Check sheet for the modelled part. Datum: model origin and axes. Units: mm. A direction names the side the tool comes from. Round coordinates to 2 decimals unless told otherwise and drop trailing zeros. Loops run counter-clockwise (first coordinate to the right, second up) from the corner with the lowest first, then second, coordinate; pieces in that order, holes last. Notation, with made-up numbers: (2, 87) - (31, 87) arc R17 cw to (31, 116) - close; hole circle Ø6 at (75, 74). An arc over 180 degrees is marked (long way). Put each result on its own line as item: value. Start each with the question number.
Item 1: Tool access check on faces 1 (the flat face through (-12.24, 16.91, 0.49)), 2 (the flat face through (2, 3, 1)), 3 (the cylindrical face through (-8.962, -15.834, 0.493)), 4 (the flat face through (-10.633, 19.445, 0.986)). Record the directions out of +Z, -Z, +X, -X, +Y, -Y that give a thin tool (end or side, any length) a straight path to the whole face; none if there is none.
Item 2: Section check B-B, the plane z = 0.35. Record the cut outline in (x, y).
Item 3: Draft check along X on faces 5 (the flat face through (2, -2, 0)), 6 (the flat face through (-10.656, -19.462, 0.986)), 7 (the cylindrical face through (-12.09, 19.06, 0.99)). Enter one of: pulls with the +X half, pulls with the -X half, needs draft (parallel to the pull), parting line crosses it, or undercut.
Item 4: Section check A-A, the plane x = 3. Record the cut outline in (y, z).
Item 5: Section check D-D, the plane y = -12. Record the cut outline in (x, z), and give its area (3 significant figures).
Item 6: Material ranges on line 1 along Y through (x, z) = (4.25, 1.7); line 2 along Y through (x, z) = (4, 1.6); line 3 along Z through (x, y) = (8, 16), recorded low to high.
Item 7: Section check C-C, the plane x = 9. Record the cut outline in (y, z).
Item 8: Gauge pin test, flat end, axial feed: pin 1 Ø1.5 at (x, y) = (8, 9) entering from +Z. Record the tip position at first contact, or that the pin passes through.
from build123d import *

# Parameters (mm, degrees)
BOSS_EXTRU_2_DEPTH      = 2
ENL_V_START             = -1
ENL_V_MAT_EXTRU_1_DEPTH = 1


with BuildPart() as part:
    # Esquisse1 → Boss.-Extru.2 (new body)
    with BuildSketch(Plane.XY):
        with BuildLine():
            Line((-12.922465041, 17.386083667), (-11.5420173, 16.419483753))
            ThreePointArc((-11.5420173, 16.419483753), (-8.998687611, 15.827772592), (-6.753604006, 17.161282102))
            ThreePointArc((-6.753604006, 17.161282102), (7.619740739, 15.766902052), (0, 3.5))
            ThreePointArc((0, 3.5), (-3.5, 0), (0, -3.5))
            ThreePointArc((0, -3.5), (7.619740739, -15.766902052), (-6.753604006, -17.161282102))
            ThreePointArc((-6.753604006, -17.161282102), (-8.998687611, -15.827772592), (-11.5420173, -16.419483753))
            Line((-11.5420173, -16.419483753), (-12.922465041, -17.386083667))
            ThreePointArc((-12.922465041, -17.386083667), (-12.266740841, -18.747374982), (-11.46812862, -20.030070109))
            Line((-11.46812862, -20.030070109), (-9.821287991, -18.876939886))
            ThreePointArc((-9.821287991, -18.876939886), (-9.457955178, -18.79240972), (-9.137228949, -18.982911079))
            ThreePointArc((-9.137228949, -18.982911079), (10.309061, -17.096396894), (0, -0.5))
            ThreePointArc((0, -0.5), (-0.5, 0), (0, 0.5))
            ThreePointArc((0, 0.5), (10.309061, 17.096396894), (-9.137228949, 18.982911079))
            ThreePointArc((-9.137228949, 18.982911079), (-9.457955178, 18.79240972), (-9.821287991, 18.876939886))
            Line((-9.821287991, 18.876939886), (-11.46812862, 20.030070109))
            ThreePointArc((-11.46812862, 20.030070109), (-12.266740841, 18.747374982), (-12.922465041, 17.386083667))
        make_face()
    extrude(amount=BOSS_EXTRU_2_DEPTH)

    # Esquisse2 → Enlèv. mat.-Extru.1 (cut)
    with BuildSketch(Plane.XY.offset(2).offset(ENL_V_START)):
        with BuildLine():
            Line((-12.922465041, 17.386083667), (-11.5420173, 16.419483753))
            ThreePointArc((-11.5420173, 16.419483753), (-8.998687611, 15.827772592), (-6.753604006, 17.161282102))
            ThreePointArc((-6.753604006, 17.161282102), (7.619740739, 15.766902052), (0, 3.5))
            ThreePointArc((0, 3.5), (-3.5, 0), (0, -3.5))
            ThreePointArc((0, -3.5), (7.619740739, -15.766902052), (-6.753604006, -17.161282102))
            ThreePointArc((-6.753604006, -17.161282102), (-8.998687611, -15.827772592), (-11.5420173, -16.419483753))
            Line((-11.5420173, -16.419483753), (-12.922465041, -17.386083667))
            Line((-12.922465041, -17.386083667), (-12.979954825, -18.647113037))
            Line((-12.979954825, -18.647113037), (-12.348888604, -18.205235712))
            Line((-12.348888604, -18.205235712), (-10.968440864, -17.238635798))
            ThreePointArc((-10.968440864, -17.238635798), (-9.1517768, -16.815984968), (-7.548145653, -17.768491761))
            ThreePointArc((-7.548145653, -17.768491761), (8.516180826, -16.210066999), (0, -2.5))
            ThreePointArc((0, -2.5), (-2.5, 0), (0, 2.5))
            ThreePointArc((0, 2.5), (8.516180826, 16.210066999), (-7.548145653, 17.768491761))
            ThreePointArc((-7.548145653, 17.768491761), (-9.1517768, 16.815984968), (-10.968440864, 17.238635798))
            Line((-10.968440864, 17.238635798), (-12.348888604, 18.205235712))
            Line((-12.348888604, 18.205235712), (-12.898926694, 18.590376529))
            Line((-12.898926694, 18.590376529), (-13.29562882, 18.205235712))
            Line((-13.29562882, 18.205235712), (-12.922465041, 17.386083667))
        make_face()
    extrude(amount=ENL_V_MAT_EXTRU_1_DEPTH, mode=Mode.SUBTRACT)


solid = part.part
Check result:
1. face 1: +Z, -Z, -X
1. face 2: +Z
1. face 3: +Z, -Z
1. face 4: +Z, -Z, +Y
2. outline: (-12.92, -17.39) arc R14 ccw to (-11.47, -20.03) - (-9.82, -18.88) arc R0.5 cw to (-9.14, -18.98) arc R11.5 ccw (long way) to (0, -0.5) arc R0.5 cw to (0, 0.5) arc R11.5 ccw (long way) to (-9.14, 18.98) arc R0.5 cw to (-9.82, 18.88) - (-11.47, 20.03) arc R14 ccw to (-12.92, 17.39) - (-11.54, 16.42) arc R3.5 ccw to (-6.75, 17.16) arc R8.5 cw (long way) to (0, 3.5) arc R3.5 ccw to (0, -3.5) arc R8.5 cw (long way) to (-6.75, -17.16) arc R3.5 ccw to (-11.54, -16.42) - close
3. face 5: needs draft
3. face 6: undercut
3. face 7: pulls with the -X half
4. outline: (-23.1, 0) - (-19.95, 0) - (-19.95, 1) - (-21.01, 1) - (-21.01, 2) - (-23.1, 2) - close; (-4.05, 0) - (-0.9, 0) - (-0.9, 2) - (-2.99, 2) - (-2.99, 1) - (-4.05, 1) - close; (0.9, 0) - (4.05, 0) - (4.05, 1) - (2.99, 1) - (2.99, 2) - (0.9, 2) - close; (19.95, 0) - (23.1, 0) - (23.1, 2) - (21.01, 2) - (21.01, 1) - (19.95, 1) - close
5. outline: (8.5, 0) - (11.5, 0) - (11.5, 2) - (9.5, 2) - (9.5, 1) - (8.5, 1) - close
5. area: 5.00 mm²
6. line 1: -22.69 to -20.5, -3.5 to -1.31, 1.31 to 3.5, 20.5 to 22.69
6. line 2: -22.78 to -20.62, -3.38 to -1.22, 1.22 to 3.38, 20.62 to 22.78
6. line 3: 0 to 1
7. outline: (-19.16, 0) - (-4.84, 0) - (-4.84, 2) - (-8.96, 2) - (-8.96, 1) - (-15.04, 1) - (-15.04, 2) - (-19.16, 2) - close; (4.84, 0) - (19.16, 0) - (19.16, 2) - (15.04, 2) - (15.04, 1) - (8.96, 1) - (8.96, 2) - (4.84, 2) - close
8. pin 1: z = 1
